Here's how the part is built. I have some questions about the finished solid (model axes, mm). A direction names the side the tool comes from. Coordinates: 2 decimals unless noted, no trailing zeros. Order: outer loops, then holes, each group sorted by start corner. A loop starts at its lowest first (then second) coordinate and runs counter-clockwise, first axis right, second up. Notation, with made-up numbers: M 75,13.5 L 130,13.5 A19 cw 130,31.5 Z; hole C 52,17 d10. An arc over 180 degrees is marked long. One line per question, with ' | ' between items. Start each with the question number.
```python
from build123d import *

# Parameters (mm, degrees)
F0_W     = 76.2
F0_H     = 63.5
F0_R     = 5.08
F0_R_2   = 6.35
F1_DEPTH = 25.4
F2_R     = 5.08
F3_R     = 7.4676
F3_R_2   = 5.08
F4_DEPTH = 6.35


with BuildPart() as f1:
    # F0 (on Front) → F1 (new body)
    with BuildSketch(Plane.XZ):
        Rectangle(F0_W, F0_H)
        with Locations((0, -15.24)):
            Circle(F0_R, mode=Mode.SUBTRACT)
        with Locations((-15.24, 0)):
            Circle(F0_R, mode=Mode.SUBTRACT)
        Circle(F0_R_2, mode=Mode.SUBTRACT)
        with Locations((15.24, 0)):
            Circle(F0_R, mode=Mode.SUBTRACT)
        with Locations((0, 15.24)):
            Circle(F0_R, mode=Mode.SUBTRACT)
    extrude(amount=F1_DEPTH)

    # F2
    f2_edges = [f1.edges().sort_by_distance(p)[0] for p in [
        (0, -25.4, 31.75),
        (-38.1, -25.4, 0),
        (0, -25.4, -31.75),
        (38.1, -25.4, 0),
    ]]
    fillet(f2_edges, radius=F2_R)

    # F3 (on face) → F4 (cut)
    with BuildSketch(Plane.XZ.offset(25.4)):
        with Locations((-15.24, 0)):
            Circle(F3_R)
        with Locations((0, 15.24)):
            Circle(F3_R)
        with Locations((15.24, 0)):
            Circle(F3_R)
        with Locations((0, -15.24)):
            Circle(F3_R)
        with Locations((0, -15.24)):
            Circle(F3_R_2)
        with Locations((-15.24, 0)):
            Circle(F3_R_2)
        with Locations((0, 15.24)):
            Circle(F3_R_2)
        with Locations((15.24, 0)):
            Circle(F3_R_2)
    extrude(amount=-F4_DEPTH, mode=Mode.SUBTRACT)


solid = f1.part
```
1. I need wall thicknesses on line 1 (Z direction, x = 0, y = -6.75); line 2 (Z direction, x = 15.24, y = -10.5); line 3 (X direction, y = -9.75, z = -0.5). Which ranges of each line are inside material? Lowest first, please.
2. Imagine slicing it at D-D (z = 0). List the corners of the cut face in (x, y) for me, then the cut area to 3 significant figures.
3. Will these pins go through, and if not, where does the flat tip stop? pin 1 (12 mm diameter, centred on x = -15.24, z = 0, fed in from -Y); pin 2 (9 mm diameter, centred on x = -15.24, z = 0, fed in from +Y) (3 decimals).
4. Imagine slicing it at A-A (z = 15.24). List the corners of the cut face in (x, y) for me.
5. Which directions (+Z, -Z, +X, -X, +Y, -Y) give clear straight access to the entire face, cutting with the end or side of a thin tool? Please do faces 1 (the face through (38.1, -10, 0)), 2 (the face through (5, -19.05, -17)).
6. We'd pull the mould along X, two halves only. Please class faces 3 (the face through (14.579, -9.392, 5.037)), 4 (the face through (0.533, -23.872, -30.301)), 5 (the face through (-38.1, -10, 0)): released by +X, released by -X, zero draft, split by the parting line, or undercut.
7. Imagine slicing it at C-C (y = -9). List the corners of the cut face in (x, z) for me, then the cut area to 3 significant figures.
8. Imagine slicing it at B-B (x = -15.24). List the corners of the cut face in (y, z) for me.
Entries:
1) line 1: -31.75 to -20.32, -10.16 to -6.35, 6.35 to 10.16, 20.32 to 31.75 | line 2: -31.75 to -5.08, 5.08 to 31.75 | line 3: -38.1 to -20.3, -10.18 to -6.33, 6.33 to 10.18, 20.3 to 38.1
2) outline: M -38.1,-20.32 A5.08 ccw -33.02,-25.4 L -22.71,-25.4 L -22.71,-19.05 L -20.32,-19.05 L -20.32,0 L -38.1,0 Z; M -10.16,-19.05 L -7.77,-19.05 L -7.77,-25.4 L -6.35,-25.4 L -6.35,0 L -10.16,0 Z; M 6.35,-25.4 L 7.77,-25.4 L 7.77,-19.05 L 10.16,-19.05 L 10.16,0 L 6.35,0 Z; M 20.32,-19.05 L 22.71,-19.05 L 22.71,-25.4 L 33.02,-25.4 A5.08 ccw 38.1,-20.32 L 38.1,0 L 20.32,0 Z | area: 1,030 mm²
3) pin 1: y = -19.05 | pin 2: through
4) outline: M -38.1,-20.32 A5.08 ccw -33.02,-25.4 L -7.47,-25.4 L -7.47,-19.05 L -5.08,-19.05 L -5.08,0 L -38.1,0 Z; M 5.08,-19.05 L 7.47,-19.05 L 7.47,-25.4 L 33.02,-25.4 A5.08 ccw 38.1,-20.32 L 38.1,0 L 5.08,0 Z
5) face 1: +Z, -Z, +X, +Y, -Y | face 2: -Y
6) face 3: undercut | face 4: zero draft | face 5: released by -X
7) outline: M -38.1,-31.75 L 38.1,-31.75 L 38.1,31.75 L -38.1,31.75 Z; hole C -15.24,0 d10.16; hole C 0,0 d12.7; hole C 0,-15.24 d10.16; hole C 0,15.24 d10.16; hole C 15.24,0 d10.16 | area: 4,390 mm²
8) outline: M -25.4,-26.67 A5.08 ccw -20.32,-31.75 L 0,-31.75 L 0,-5.08 L -19.05,-5.08 L -19.05,-7.47 L -25.4,-7.47 Z; M -25.4,7.47 L -19.05,7.47 L -19.05,5.08 L 0,5.08 L 0,31.75 L -20.32,31.75 A5.08 ccw -25.4,26.67 Z
